Can you work these out from the model? Positions are in its coordinate system, mm. A direction names the side the tool comes from. Give positions to 0.01 mm unless a question says otherwise; leave off trailing zeros. Order: outer loops, then holes, each group sorted by start corner. A loop starts at its lowest first (then second) coordinate and runs counter-clockwise, first axis right, second up. Notation, with made-up numbers: M -12,55.25 L 17,55.25 A16 cw 17,73.25 Z; hole C 19.25,-14 d11. An arc over 180 degrees is marked long. Use a Markdown table: item, result. Add a question column.
from build123d import *

# Parameters (mm, degrees)
SKETCH1_R           = 1.5
SKETCH1_R_2         = 53.34
BOSS_EXTRUDE1_DEPTH = 3.175
CUT_EXTRUDE3_DEPTH  = 140.736059076
CUT_EXTRUDE4_DEPTH  = 140.736059076
CUT_EXTRUDE5_DEPTH  = 140.736059076
SKETCH6_R           = 1.5
CUT_EXTRUDE6_DEPTH  = 130.738840902


with BuildPart() as part:
    # Sketch1 → Boss-Extrude1 (new body)
    with BuildSketch(Plane(origin=(0, 0, 0), x_dir=(1, 0, 0), z_dir=(0, 1, 0))):
        Polygon((0.047005036, -98.782806148), (-98.782806148, -0.047005036), (-0.047005036, 98.782806148), (98.782806148, 0.047005036), align=None)
        with Locations(Location((-61.346730494, 5.55625, 0), (0, 0, 270))):
            Circle(SKETCH1_R, mode=Mode.SUBTRACT)
        with Locations(Location((-61.346730494, -5.55625, 0), (0, 0, 270))):
            Circle(SKETCH1_R, mode=Mode.SUBTRACT)
        with Locations(Location((-5.55625, -61.346730494, 0), (0, 0, 270))):
            Circle(SKETCH1_R, mode=Mode.SUBTRACT)
        with Locations(Location((5.55625, -61.346730494, 0), (0, 0, 270))):
            Circle(SKETCH1_R, mode=Mode.SUBTRACT)
        with Locations(Location((61.346730494, -5.55625, 0), (0, 0, 270))):
            Circle(SKETCH1_R, mode=Mode.SUBTRACT)
        with Locations(Location((61.346730494, 5.55625, 0), (0, 0, 270))):
            Circle(SKETCH1_R, mode=Mode.SUBTRACT)
        with Locations(Location((5.55625, 61.346730494, 0), (0, 0, 270))):
            Circle(SKETCH1_R, mode=Mode.SUBTRACT)
        with Locations(Location((-5.55625, 61.346730494, 0), (0, 0, 270))):
            Circle(SKETCH1_R, mode=Mode.SUBTRACT)
        with Locations(Location((0, 0, 0), (0, 0, 270))):
            Circle(SKETCH1_R_2, mode=Mode.SUBTRACT)
    extrude(amount=BOSS_EXTRUDE1_DEPTH)

    # Sketch2 → Cut-Extrude3 (cut, through all)
    with BuildSketch(Plane(origin=(0, 3.175, 0), x_dir=(1, 0, 0), z_dir=(0, 1, 0))):
        Polygon((3.175, 53.34), (3.175, 59.69), (-3.175, 59.69), (-3.175, 53.34), (-3.175, 52.244537665), (3.175, 52.244537665), align=None)
        Polygon((53.34, -3.175), (59.69, -3.175), (59.69, 3.175), (53.34, 3.175), (52.244537665, 3.175), (52.244537665, -3.175), align=None)
        Polygon((-3.175, -53.34), (-3.175, -59.69), (3.175, -59.69), (3.175, -53.34), (3.175, -52.244537665), (-3.175, -52.244537665), align=None)
        Polygon((-53.34, 3.175), (-59.69, 3.175), (-59.69, -3.175), (-53.34, -3.175), (-52.244537665, -3.175), (-52.244537665, 3.175), align=None)
    extrude(amount=-CUT_EXTRUDE3_DEPTH, mode=Mode.SUBTRACT)

    # Sketch3 → Cut-Extrude4 (cut, through all)
    with BuildSketch(Plane(origin=(0, 3.175, 0), x_dir=(1, 0, 0), z_dir=(0, 1, 0))):
        Polygon((-49.414905592, 49.367900556), (49.414905592, -49.367900556), (0.047005036, -98.782806148), (-98.782806148, -0.047005036), align=None)
    extrude(amount=-CUT_EXTRUDE4_DEPTH, mode=Mode.SUBTRACT)

    # Sketch5 → Cut-Extrude5 (cut, through all)
    with BuildSketch(Plane(origin=(0, 3.175, 0), x_dir=(1, 0, 0), z_dir=(0, 1, 0))):
        Polygon((98.782806148, 0.047005036), (91.71510385, -7.027426688), (-7.114707335, 91.708374424), (-0.047005036, 98.782806148), align=None)
    extrude(amount=-CUT_EXTRUDE5_DEPTH, mode=Mode.SUBTRACT)

    # Sketch6 → Cut-Extrude6 (cut, through all)
    with BuildSketch(Plane(origin=(0, 3.175, 0), x_dir=(1, 0, 0), z_dir=(0, 1, 0))):
        with Locations(Location((64.725061333, -22.363275374, 0), (0, 0, 270))):
            Circle(SKETCH6_R)
        with Locations(Location((75.300110897, -11.778156907, 0), (0, 0, 270))):
            Circle(SKETCH6_R)
        with Locations(Location((-12.105083926, 74.865628777, 0), (0, 0, 90))):
            Circle(SKETCH6_R)
        with Locations(Location((-22.597274037, 64.198372666, 0), (0, 0, 90))):
            Circle(SKETCH6_R)
        with Locations(Location((54.150011768, -32.948393841, 0), (0, 0, 270))):
            Circle(SKETCH6_R)
        with Locations(Location((-33.089464147, 53.531116555, 0), (0, 0, 90))):
            Circle(SKETCH6_R)
    extrude(amount=-CUT_EXTRUDE6_DEPTH, mode=Mode.SUBTRACT)


solid = part.part
1. If we section it at A-A, the plane z = -47: List the corners of the cut face in (x, y) for me (3 decimals).
2. If we section it at B-B, the plane y = 0.7: State how many separate pieces and enclosed holes the cut face has, then the cut area to 3 significant figures.
3. If we section it at D-D, the plane z = 17.5: List the corners of the cut face in (x, y) for me (1 decimal), then the cut area to 3 significant figures.
4. Will these pins go through, and if not, where does the flat tip stop? pin 1 (5 mm diameter, centred on x = -33.09, z = -53.53, fed in from -Y); pin 2 (1 mm diameter, centred on y = 1, z = -77, fed in from -X); pin 3 (1.6 mm diameter, centred on y = 2, z = -57.5, fed in from -X); pin 4 (2.5 mm diameter, centred on x = 64.73, z = 22.36, fed in from -Y).
5. If we section it at C-C, the plane x = 27: List the corners of the cut face in (y, z) for me (3 decimals), then the cut area to 3 significant figures.
6. We'd pull the mould along X, two halves only. Please class faces 4 (the face through (43.49, 1.61, 43.45)), 5 (the face through (70.86, 1.57, 27.9)), 6 (the face through (-3.175, 2, -57)), 7 (the face through (37, 3.175, -42)): +X half, -X half, draft (parallel to the pull), parting line (faces both ways), or undercut.
7. On a 3-axis mill with a long thin cutter (end or side, diameter ignored), from which of +Z, -Z, +X, -X, +Y, -Y can I reach the whole of each face in a straight line? I mean faces 1 (the face through (38.1, 1.57, -37.33)), 2 (the face through (57, 2, -3.175)), 3 (the face through (0, 2, -59.69)). Say none if no direction works.
8. I need wall thicknesses on L1, parallel to Z at x = 49, y = 1.35 (3 decimals); L2, parallel to X at y = 0.55, z = 21.5; L3, parallel to Z at x = 58, y = 2.55 (3 decimals). Which ranges of each line are inside material? Lowest first, please. Write a range as [from, to].
Geometry results:
| question | item | result |
|---|---|---|
| 1 | outline | M -47.045,0 L -25.222,0 L -25.222,3.175 L -47.045,3.175 Z; M 25.222,0 L 37.636,0 L 37.636,3.175 L 25.222,3.175 Z |
| 2 | separate pieces | 1 |
| 2 | enclosed holes | 10 |
| 2 | area | 3,740 mm^2 |
| 3 | outline | M 50.4,0 L 81.3,0 L 81.3,3.2 L 50.4,3.2 Z |
| 3 | area | 98.0 mm^2 |
| 4 | pin 1 | stops at y = 0 |
| 4 | pin 2 | stops at x = -22.31 |
| 4 | pin 3 | stops at x = -42.09 |
| 4 | pin 4 | passes through |
| 5 | outline | M 0,-57.626 L 3.175,-57.626 L 3.175,-46.002 L 0,-46.002 Z |
| 5 | area | 36.9 mm^2 |
| 6 | face 4 | -X half |
| 6 | face 5 | +X half |
| 6 | face 6 | undercut |
| 6 | face 7 | draft |
| 7 | face 1 | +Y, -Y |
| 7 | face 2 | -X, +Y, -Y |
| 7 | face 3 | +Z, +Y, -Y |
| 8 | L1 | z = [-35.647, -21.075], [21.075, 48.953] |
| 8 | L2 | x = [48.82, 63.5], [65.95, 77.26] |
| 8 | L3 | z = [-26.656, -3.175], [3.175, 40.775] |
